Build history of the part. All positions in model axes, mm. A direction names the side the tool comes from. Give positions to 0.01 mm unless a question says otherwise; leave off trailing zeros. Loops run counter-clockwise (first coordinate to the right, second up) from the corner with the lowest first, then second, coordinate; pieces in that order, holes last. Notation, with made-up numbers: (70, 83) - (117, 83) arc R34 cw to (117, 117) - close; hole circle Ø3 at (19.25, 70). An arc over 180 degrees is marked (long way). Return JSON: item names as keys, results as strings. Group by question number.
1) Mould opens along Y. For faces 6 (the face through (12.5, 105.137, -26.3)), 7 (the face through (13, 117.837, -11)), 8 (the face through (13.389, 63.933, -6.439)), 9 (the face through (9.6, 111.58, -23.55)) say: released by +Y, released by -Y, zero draft, split by the parting line, or undercut.
2) Drop flat-ended pins along their axis: pin 1 (6.5 mm diameter, centred on x = 15, y = 66, fed in from +Z); pin 2 (5 mm diameter, centred on x = 15, z = 15, fed in from +Y); pin 3 (16.5 mm diameter, centred on x = 12.7, y = 35.29, fed in from +Z); pin 4 (5 mm diameter, centred on x = 34.925, z = 38.1, fed in from +Y). Give the stop position or say it passes through.
3) Drill centre lines: probe 1 along Y at (x, z) = (12, -11); probe 2 along X at (y, z) = (-113.25, 12.7); probe 3 along Y at (x, z) = (12.7, -9.5). Where is each one in solid material? Low to high. Write a range as from..to.
4) Slice it at B-B (z = 18). List the corners of the cut face in (x, y).
5) Slice it at A-A (z = -22.86). List the corners of the cut face in (x, y) (3 decimals).
6) Slice it at C-C (x = 28). List the corners of the cut face in (y, z), and give its area (3 significant figures).
7) 3-axis set-ups, long thin cutter, end or side, ignore diameter. For faces 1 (the face through (13, -8, -12.7)), 2 (the face through (10.79, 60.98, 11.39)), 3 (the face through (35, -105.137, 23)), 4 (the face through (26.853, -113.789, -12.268)), 5 (the face through (38.073, -111.576, 13.113)): which of +Z, -Z, +X, -X, +Y, -Y reach the whole face in a straight line?
8) Slice it at D-D (z = 38.1). List the corners of the cut face in (x, y), and give its area (3 significant figures).
```python
from build123d import *

# Parameters (mm, degrees)
SKETCH3_W           = 38.1
SKETCH3_H           = 12.7
SKETCH3_W_2         = 19.05
BOSS_EXTRUDE1_DEPTH = 25.4
FILLET1_R           = 6.35
FILLET3_R           = 2.54
SKETCH9_R           = 3.175
CUT_EXTRUDE2_DEPTH  = 243.42109467
SKETCH10_R          = 3.225000027
SKETCH10_R_2        = 3.180000003
CUT_EXTRUDE3_DEPTH  = 137.245942271
SKETCH18_R          = 6.35
CUT_EXTRUDE4_DEPTH  = 38.1
SKETCH19_W          = 19.05
SKETCH19_H          = 63.5
SKETCH19_R          = 3.175
BOSS_EXTRUDE4_DEPTH = 12.7
FILLET6_R           = 2.54
FILLET7_R           = 6.35


with BuildPart() as part:
    # Sketch3 → Boss-Extrude1 (new body)
    with BuildSketch(Plane(origin=(0, 0, 0), x_dir=(0, 0, -1), z_dir=(1, 0, 0))):
        Polygon((-12.7, -105.13695), (-12.7, -117.83695), (12.7, -117.83695), (12.7, 105.13695), (12.7, 117.83695), (-12.7, 117.83695), (-50.8, -105.13695), align=None)
        with Locations((-31.75, -111.48695)):
            Rectangle(SKETCH3_W, SKETCH3_H)
        with Locations((22.225, 111.48695)):
            Rectangle(SKETCH3_W_2, SKETCH3_H)
    extrude(amount=BOSS_EXTRUDE1_DEPTH)

    # Fillet1
    fillet1_edges = [part.edges().sort_by_distance(p)[0] for p in [
        (12.7, 105.13695, -12.7),
        (12.7, -117.83695, -12.7),
        (12.7, 117.83695, 12.7),
    ]]
    fillet(fillet1_edges, radius=FILLET1_R)

    # Fillet3
    fillet3_edges = [part.edges().sort_by_distance(p)[0] for p in [
        (12.7, 117.83695, -31.75),
        (12.7, 105.13695, -31.75),
        (12.7, -117.83695, 50.8),
    ]]
    fillet(fillet3_edges, radius=FILLET3_R)

    # Sketch9 → Cut-Extrude2 (cut, through all)
    with BuildSketch(Plane(origin=(0, 117.83695, 0), x_dir=(1, 0, 0), z_dir=(0, 1, 0))):
        with Locations(Location((12.7, 22.86, 0), (0, 0, 270))):
            Circle(SKETCH9_R)
    extrude(amount=-CUT_EXTRUDE2_DEPTH, mode=Mode.SUBTRACT)

    # Sketch10 → Cut-Extrude3 (cut, through all)
    with BuildSketch(Plane(origin=(0, 0, -12.7), x_dir=(-1, 0, 0), z_dir=(0, 0, -1))):
        with Locations((-12.7, 35.28695)):
            Circle(SKETCH10_R)
        with Locations((-12.7, 67.03695)):
            Circle(SKETCH10_R_2)
    extrude(amount=-CUT_EXTRUDE3_DEPTH, mode=Mode.SUBTRACT)

    # Sketch18 → Cut-Extrude4 (cut)
    with BuildSketch(Plane(origin=(0, 0, 38.1), x_dir=(-1, 0, 0), z_dir=(0, 0, -1))):
        with Locations(Location((-12.7, 67.03695, 0), (0, 0, 270))):
            Circle(SKETCH18_R)
        with Locations(Location((-12.7, 35.28695, 0), (0, 0, 270))):
            Circle(SKETCH18_R)
    extrude(amount=CUT_EXTRUDE4_DEPTH, mode=Mode.SUBTRACT)

    # Sketch19 → Boss-Extrude4 (add)
    with BuildSketch(Plane.XZ.offset(117.83695)):
        with Locations((34.925, 19.05)):
            Rectangle(SKETCH19_W, SKETCH19_H)
        with Locations(Location((34.925, 38.1, 0), (0, 0, 270))):
            Circle(SKETCH19_R, mode=Mode.SUBTRACT)
        with Locations(Location((34.925, 12.7, 0), (0, 0, 270))):
            Circle(SKETCH19_R, mode=Mode.SUBTRACT)
    extrude(amount=-BOSS_EXTRUDE4_DEPTH)

    # Fillet6
    fillet6_edges = [part.edges().sort_by_distance(p)[0] for p in [
        (34.925, -117.83695, 50.8),
    ]]
    fillet(fillet6_edges, radius=FILLET6_R)

    # Fillet7
    # the kernel refuses this fillet: 6.35 mm, written as the material it takes off along each edge
    with BuildSketch(Plane(origin=(9.525, -117.83695, -12.7), x_dir=(0, 0, 1), z_dir=(1, 0, 0))) as fillet7_piece_1:
        with BuildLine():
            CenterArc((FILLET7_R, -FILLET7_R), FILLET7_R, 90, 90)
            Line((0, -FILLET7_R), (0, 0))
            Line((0, 0), (FILLET7_R, 0))
        make_face()
    extrude(amount=50.8, mode=Mode.SUBTRACT)
    with BuildSketch(Plane(origin=(25.4, -105.13695, -12.7), x_dir=(0, 0, 1), z_dir=(1, 0, 0))) as fillet7_piece_2:
        with BuildLine():
            CenterArc((FILLET7_R, FILLET7_R), FILLET7_R, 180, 90)
            Line((0, FILLET7_R), (0, 0))
            Line((0, 0), (FILLET7_R, 0))
        make_face()
    extrude(amount=34.925, mode=Mode.SUBTRACT)


solid = part.part
```
Results:
{
 "1": {"face 6": "released by -Y", "face 7": "released by +Y", "face 8": "undercut", "face 9": "zero draft"},
 "2": {"pin 1": "z = 0", "pin 2": "y = 115.19", "pin 3": "z = 28.21", "pin 4": "through"},
 "3": {"probe 1": "-115.81..32.14, 38.44..63.93, 70.14..117.84", "probe 2": "0..31.75, 38.1..44.45", "probe 3": "-117..32.06, 38.51..63.86, 70.22..117.84"},
 "4": {"outline": "(0, -117.84) - (44.45, -117.84) - (44.45, -105.14) - (25.4, -105.14) - (25.4, 86.82) - (0, 86.82) - close; hole circle Ø12.7 at (12.7, 35.29); hole circle Ø12.7 at (12.7, 67.04)"},
 "5": {"outline": "(0, 105.137) - (9.525, 105.137) - (9.525, 117.837) - (0, 117.837) - close; (15.875, 105.137) - (25.4, 105.137) - (25.4, 117.837) - (15.875, 117.837) - close"},
 "6": {"outline": "(-117.84, -6.35) arc R6.35 ccw to (-105.14, -6.35) - (-105.14, 50.8) - (-115.3, 50.8) arc R2.54 ccw to (-117.84, 48.26) - close", "area": "788 mm2"},
 "7": {"face 1": "-Z, +X, -X, -Y", "face 2": "+Z", "face 3": "+Z, -Z, +X, +Y", "face 4": "-Z, +X", "face 5": "+Y, -Y"},
 "8": {"outline": "(0, -117.84) - (31.75, -117.84) - (31.75, -105.14) - (25.4, -105.14) - (25.4, -30.81) - (0, -30.81) - close; (38.1, -117.84) - (44.45, -117.84) - (44.45, -105.14) - (38.1, -105.14) - close", "area": "2,370 mm2"}
}
